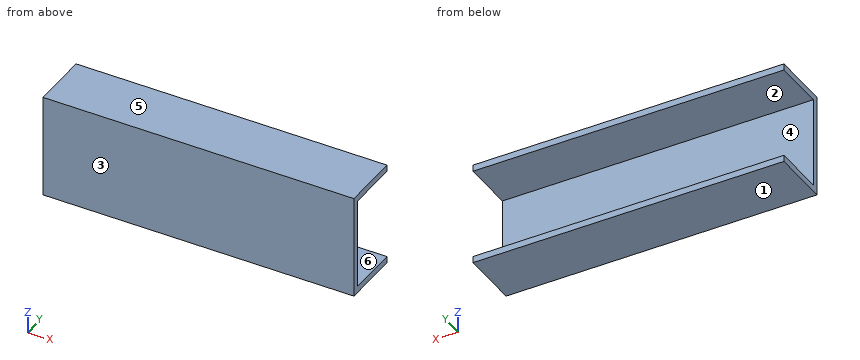
from build123d import *

# Parameters (mm, degrees)
F0_W     = 304.8
F0_H     = 101.6
F1_DEPTH = 6.35
F2_W     = 304.8
F2_H     = 6.35
F3_DEPTH = 50.8
F4_DEPTH = 50.8


with BuildPart() as f1:
    # F0 (on Front) → F1 (new body)
    with BuildSketch(Plane.XZ):
        with Locations((19.505125, -12.510431)):
            Rectangle(F0_W, F0_H)
    extrude(amount=F1_DEPTH)

    # F2 (on face) → F3 (join)
    with BuildSketch(Plane(origin=(0, 0, 0), x_dir=(-1, 0, 0), z_dir=(0, 1, 0))):
        with Locations((-19.505125, 35.114569)):
            Rectangle(F2_W, F2_H)
    extrude(amount=F3_DEPTH)

    # F2 (on face) → F4 (join)
    with BuildSketch(Plane(origin=(0, 0, 0), x_dir=(-1, 0, 0), z_dir=(0, 1, 0))):
        with Locations((-19.505125, -60.135431)):
            Rectangle(F2_W, F2_H)
    extrude(amount=F4_DEPTH)


solid = f1.part
Input: part model. Units: mm. Frame: model coordinates. Face numbers are marked on the shaded views. A direction names the side the tool comes from. Coordinates: 2 decimals unless noted, no trailing zeros. Order: outer loops, then holes, each group sorted by start corner. A loop starts at its lowest first (then second) coordinate and runs counter-clockwise, first axis right, second up.
1. Cut plane C-C, the plane z = -46.5. Return loops of the section in (x, y), plus the area to 3 significant figures.
Checked values:
outline: (-132.89, -6.35) - (171.91, -6.35) - (171.91, 0) - (-132.89, 0) - close
area: 1,940 mm2
2. Ray query, line 1 along Z through (x, y) = (-51, 4.5); line 2 along Y through (x, z) = (141, -51). Return the intervals inside material, ascending.
Checked values:
line 1: z = -63.31 to -56.96, 31.94 to 38.29
line 2: y = -6.35 to 0
3. Cut plane B-B, the plane x = 101. Return loops of the section in (y, z).
Checked values:
outline: (-6.35, -63.31) - (50.8, -63.31) - (50.8, -56.96) - (0, -56.96) - (0, 31.94) - (50.8, 31.94) - (50.8, 38.29) - (-6.35, 38.29) - close
4. Access query for the marked faces 5 and 6. Directions: +Z, -Z, +X, -X, +Y, -Y. A direction counts if a zero-diameter tool reaches every point of the face in a straight line with its end or side. Return the directions, or none.
Checked values:
face 5: +Z, +X, -X, +Y, -Y
face 6: +X, -X, +Y
5. Contact query for a flat-ended pin moving along its axis: P1, Ø8, axis at x = 76.5, z = 27.5, coming from the +Y side. Output: stop coordinate, or through.
Checked values:
P1: stops at y = 0
6. Draft query along Z for the marked faces 1, 2, 3 and 4. Return one class per face: +Z half, -Z half, draft (parallel to the pull), parting line (faces both ways), or undercut.
Checked values:
face 1: -Z half
face 2: undercut
face 3: draft
face 4: undercut
7. Cut plane A-A, the plane y = 20.5. Return loops of the section in (x, z), plus the area to 3 significant figures.
Checked values:
outline: (-132.89, -63.31) - (171.91, -63.31) - (171.91, -56.96) - (-132.89, -56.96) - close; (-132.89, 31.94) - (171.91, 31.94) - (171.91, 38.29) - (-132.89, 38.29) - close
area: 3,870 mm2
